Can you work these out from the model? Positions are in its coordinate system, mm. Give positions to 0.01 mm unless a question says otherwise; leave off trailing zeros. Write each loop counter-clockwise with the first axis right and the second up, starting at its lowest first coordinate (ties: lowest second). Pieces come first, ordered by that corner, then holes. Notation, with made-up numbers: (-8, 15) -> (49, 15) arc R11 cw to (49, 30) -> close; hole circle Ø3 at (63, 24). An arc over 180 degrees is marked (long way). Answer as CSV lines item,"result". Start each with the question number.
1. I'm going to push a flat-ended pin straight in: P1, Ø1, axis at x = 5.5, z = 0.5, coming from the +Y side. Where does the tip first touch, or does it pass through?
2. I need wall thicknesses on line 1 (Y direction, x = 17, z = 0.5); line 2 (X direction, y = 77.5, z = 1.75); line 3 (Y direction, x = -29, z = 0.9). Which ranges of each line are inside material? Lowest first, please. Write a range as [from, to].
3. If we section it at C-C on x = -31: Write out the boundary of the cut face in (y, z), plus the area to 3 significant figures.
4. If we section it at B-B on y = 3: Write out the boundary of the cut face in (x, z).
```python
from build123d import *

# Parameters (mm, degrees)
SKETCH_1_R      = 3
EXTRUDE_1_DEPTH = 2


with BuildPart() as part:
    # 草图1 → 凸台-拉伸1 (new body)
    with BuildSketch(Plane.XY):
        with BuildLine():
            Line((0, 57.5), (6, 67.892304845))
            ThreePointArc((6, 67.892304845), (20.196152423, 80.480762114), (16.392304845, 61.892304845))
            Line((16.392304845, 61.892304845), (6.915077614, 45.477265766))
            ThreePointArc((6.915077614, 45.477265766), (-37.990130297, 25.937424699), (-39.837168574, -23))
            ThreePointArc((-39.837168574, -23), (-41.941814646, -30.854646072), (-49.796460718, -28.75))
            ThreePointArc((-49.796460718, -28.75), (-49.796460718, 28.75), (0, 57.5))
        make_face()
        with Locations((15.196152423, 71.820508076)):
            Circle(SKETCH_1_R, mode=Mode.SUBTRACT)
    extrude(amount=EXTRUDE_1_DEPTH)


solid = part.part
```
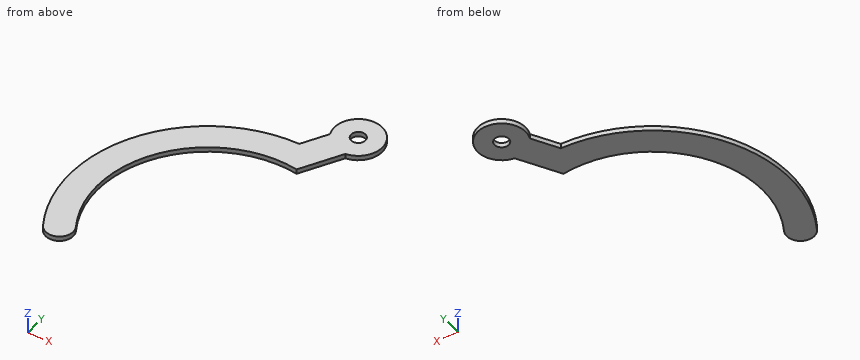
Computed values:
1,P1,"stops at y = 75.75"
2,line 1,"y = [61.98, 69.42], [74.22, 81.66]"
2,line 2,"x = [6.97, 23.43]"
2,line 3,"y = [35.71, 49.65]"
3,outline,"(33.99, 0) -> (48.43, 0) -> (48.43, 2) -> (33.99, 2) -> close"
3,area,"28.9 mm2"
4,outline,"(-57.42, 0) -> (-45.9, 0) -> (-45.9, 2) -> (-57.42, 2) -> close"
